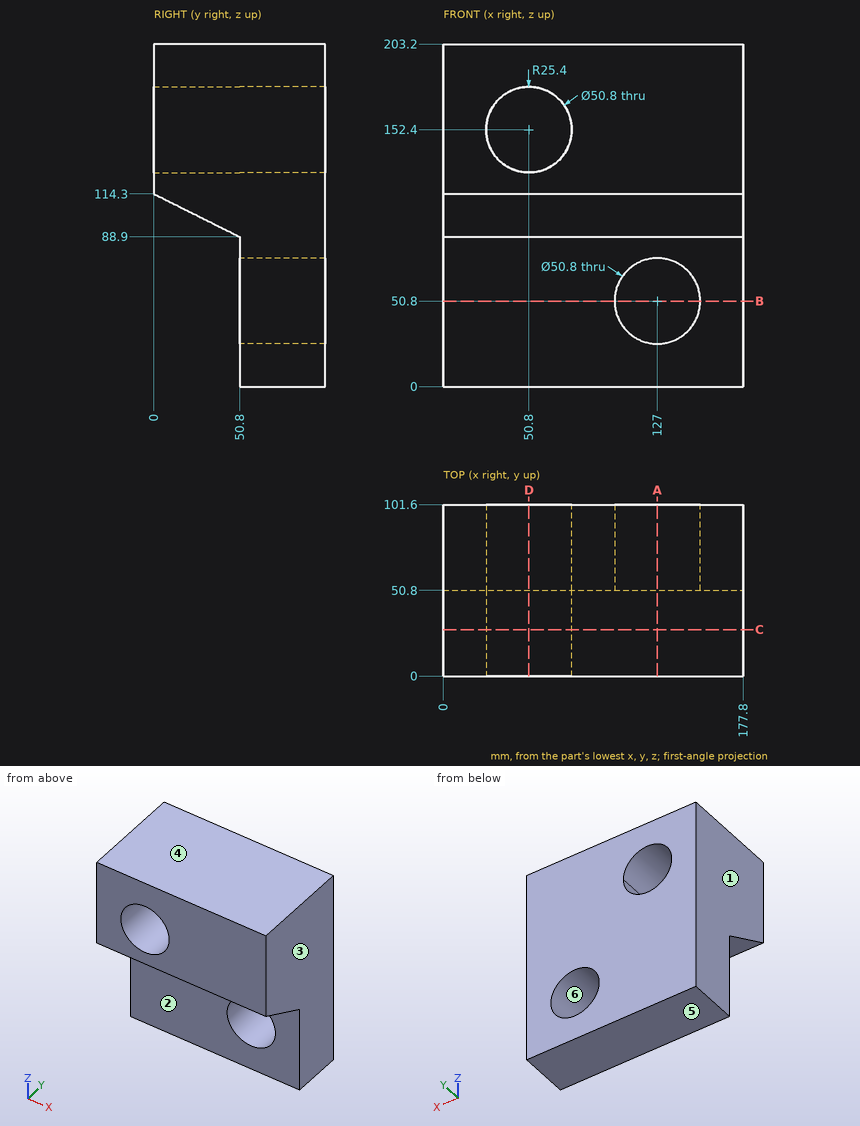
Study the drawing (mm; zero at the part's minimum x, y, z) and answer. A direction names the side the tool comes from. Coordinates: 2 decimals unless noted, no trailing zeros. Write each loop counter-clockwise with the first axis right and the second up, starting at its lowest first coordinate (ties: lowest second). Pieces come first, ordered by that corner, then holes. Notation, with made-up numbers: M 5,27 L 50,27 A17 cw 50,43 Z; hole C 83,42.25 d8. An arc over 180 degrees is marked long. Use one line per item in the form item = value.
Item 1: The mould has two halves that part along Z. Classify the marked faces 3, 4, 5 and 6: released by +Z, released by -Z, zero draft, split by the parting line, or undercut.
Model answer:
face_3 = zero draft
face_4 = released by +Z
face_5 = released by -Z
face_6 = undercut
Item 2: Find the intervals of material crossed by probe 1 along Z at (x, y) = (127, 72); probe 2 along X at (y, z) = (20, 152); probe 3 along Y at (x, z) = (50, 26.5), in increasing order.
Model answer:
probe_1 = 0 to 25.4, 76.2 to 203.2
probe_2 = 0 to 25.4, 76.2 to 177.8
probe_3 = 50.8 to 101.6
Item 3: Find section C-C, the plane y = 27.5. Give the vertices of the cut face in (x, z), plus the area to 3 significant figures.
Model answer:
outline = M 0,100.55 L 177.8,100.55 L 177.8,203.2 L 0,203.2 Z; hole C 50.8,152.4 d50.8
area = 16,200 mm2
Item 4: Find section A-A, the plane x = 127. Give the vertices of the cut face in (y, z).
Model answer:
outline = M 0,114.3 L 50.8,88.9 L 50.8,76.2 L 101.6,76.2 L 101.6,203.2 L 0,203.2 Z; M 50.8,0 L 101.6,0 L 101.6,25.4 L 50.8,25.4 Z
Item 5: Find section D-D, the plane x = 50.8. Give the vertices of the cut face in (y, z).
Model answer:
outline = M 0,114.3 L 50.8,88.9 L 50.8,0 L 101.6,0 L 101.6,127 L 0,127 Z; M 0,177.8 L 101.6,177.8 L 101.6,203.2 L 0,203.2 Z
Item 6: For the marked faces 1 and 2, determine the directions among +Z, -Z, +X, -X, +Y, -Y from which every point of the face is accessible in a straight line to the end or side of a thin tool.
Model answer:
face_1 = +Z, -Z, -X, +Y, -Y
face_2 = -Z, +X, -X, -Y
Item 7: Find section B-B, the plane z = 50.8. Give the vertices of the cut face in (x, y), plus the area to 3 significant figures.
Model answer:
outline = M 0,50.8 L 101.6,50.8 L 101.6,101.6 L 0,101.6 Z; M 152.4,50.8 L 177.8,50.8 L 177.8,101.6 L 152.4,101.6 Z
area = 6,450 mm2
Item 8: Given P1, Ø5, axis at x = 108, z = 146, coming from the -Y side; P2, Ø4, axis at x = 125, y = 15.5, coming from the -Z side; P3, Ø1, axis at x = 85.5, z = 60.5, coming from the -Y side, each flat-ended and moving along its own axis, determine where each tip first touches the part or whether it passes through.
Model answer:
P1 = 0
P2 = 105.55
P3 = 50.8
